Read the model definition and answer for the solid it produces. Units are mm, in the model's axes. Coordinates: 2 decimals unless noted, no trailing zeros. Write each loop counter-clockwise with the first axis right and the second up, starting at its lowest first coordinate (ties: lowest second). Pieces come first, ordered by that corner, then holes. Notation, with made-up numbers: (46.25, -34.5) -> (88.25, -34.5) arc R17 ccw to (88.25, -24.5) -> close; hole circle Ø11 at (65, 45.5). An arc over 180 degrees is marked (long way). Use CSV: the item, a comma, the result in double quotes.
from build123d import *

# Parameters (mm, degrees)
SKETCH_R  = 2.55
PAD_DEPTH = 37.5
FILLET_R  = 1


with BuildPart() as part:
    # Sketch → Pad (new body)
    with BuildSketch(Plane.XY):
        Polygon((-5, 0), (-2.5, -4.330127), (2.5, -4.330127), (5, 0), (2.5, 4.330127), (-2.5, 4.330127), align=None)
        Circle(SKETCH_R, mode=Mode.SUBTRACT)
    extrude(amount=PAD_DEPTH)

    # Fillet
    fillet_edges = [part.edges().sort_by_distance(p)[0] for p in [
        (-2.55, 0, 0),
    ]]
    fillet(fillet_edges, radius=FILLET_R)


solid = part.part
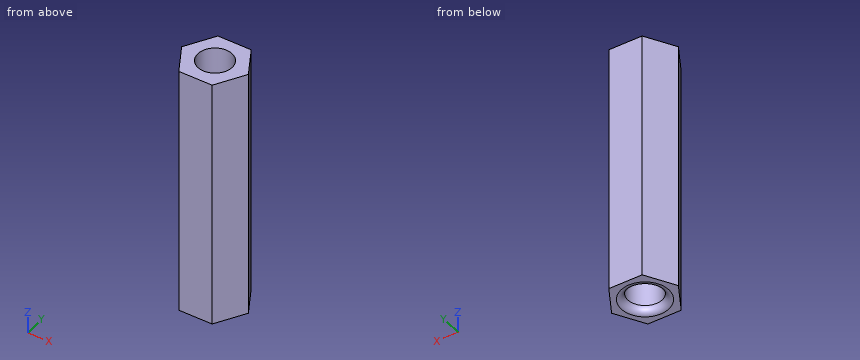
1. Each of these flat-tipped pins is pushed along its axis until it touches: pin 1 Ø4.5 at (x, y) = (0, 0) entering from -Z; pin 2 Ø1.5 at (y, z) = (2, 30) entering from -X; pin 3 Ø5 at (y, z) = (-0.5, 15.5) entering from -X; pin 4 Ø5 at (y, z) = (-3, 12) entering from -X. Where does it stop, or does it pass through?
Solutions:
pin 1,"passes through"
pin 2,"stops at x = -4.28"
pin 3,"stops at x = -5"
pin 4,"stops at x = -4.71"
2. A cutting plane is placed at B-B (z = 22). Give the vertices of the cut face in (x, y), and give its area (3 significant figures).
Solutions:
outline,"(-5, 0) -> (-2.5, -4.33) -> (2.5, -4.33) -> (5, 0) -> (2.5, 4.33) -> (-2.5, 4.33) -> close; hole circle Ø5.1 at (0, 0)"
area,"44.5 mm^2"
3. Find the intervals of material crossed by line 1 along Y through (x, z) = (-0.5, 35); line 2 along X through (y, z) = (-0.5, 11); line 3 along Y through (x, z) = (-1.5, 18.5), in increasing order.
Solutions:
line 1,"y = -4.33 to -2.5, 2.5 to 4.33"
line 2,"x = -4.71 to -2.5, 2.5 to 4.71"
line 3,"y = -4.33 to -2.06, 2.06 to 4.33"
4. A cutting plane is placed at A-A (x = 0). Give the vertices of the cut face in (y, z).
Solutions:
outline,"(-4.33, 0) -> (-3.55, 0) arc R1 ccw to (-2.55, 1) -> (-2.55, 37.5) -> (-4.33, 37.5) -> close; (2.55, 1) arc R1 ccw to (3.55, 0) -> (4.33, 0) -> (4.33, 37.5) -> (2.55, 37.5) -> close"
5. A cutting plane is placed at C-C (x = 4.25). Give the vertices of the cut face in (y, z).
Solutions:
outline,"(-1.3, 0) -> (1.3, 0) -> (1.3, 37.5) -> (-1.3, 37.5) -> close"
